Read the model definition and answer for the solid it produces. Units are mm, in the model's axes. Coordinates: 2 decimals unless noted, no trailing zeros. Order: outer loops, then holes, each group sorted by start corner. A loop starts at its lowest first (then second) coordinate and runs counter-clockwise, first axis right, second up.
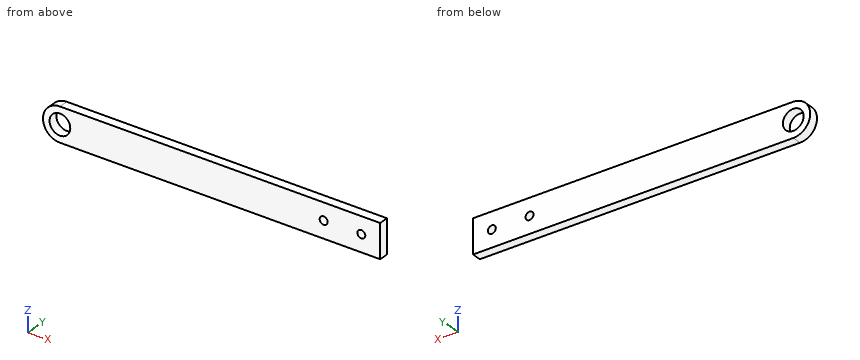
from build123d import *

# Parameters (mm, degrees)
BOSS_EXTRUDE1_DEPTH = 5
SKETCH4_R           = 2.1
CUT_EXTRUDE2_DEPTH  = 180.972220079
SKETCH5_R           = 5.5
CUT_EXTRUDE3_DEPTH  = 180.972220079


with BuildPart() as part:
    # Sketch1 → Boss-Extrude1 (new body)
    with BuildSketch(Plane(origin=(0, 0, 0), x_dir=(1, 0, 0), z_dir=(0, 1, 0))):
        with BuildLine():
            Line((0, 0), (-170, 0))
            ThreePointArc((-170, 0), (-179, -9), (-170, -18))
            Line((-170, -18), (0, -18))
            Line((0, -18), (0, 0))
        make_face()
    extrude(amount=BOSS_EXTRUDE1_DEPTH)

    # Sketch4 → Cut-Extrude2 (cut, through all)
    with BuildSketch(Plane(origin=(0, 5, 0), x_dir=(1, 0, 0), z_dir=(0, 1, 0))):
        with Locations(Location((-10, -9, 0), (0, 0, 270))):
            Circle(SKETCH4_R)
        with Locations(Location((-30, -9, 0), (0, 0, 270))):
            Circle(SKETCH4_R)
    extrude(amount=-CUT_EXTRUDE2_DEPTH, mode=Mode.SUBTRACT)

    # Sketch5 → Cut-Extrude3 (cut, through all)
    with BuildSketch(Plane(origin=(0, 5, 0), x_dir=(1, 0, 0), z_dir=(0, 1, 0))):
        with Locations(Location((-170, -9, 0), (0, 0, 270))):
            Circle(SKETCH5_R)
    extrude(amount=-CUT_EXTRUDE3_DEPTH, mode=Mode.SUBTRACT)


solid = part.part
Q1. The part is cut by section C-C, the plane z = 9. Determine the outline of the cut face in (x, y), then the cut area to 3 significant figures.
Q2. The part is cut by section B-B, the plane y = 3.5. Determine the outline of the cut face in (x, z).
Q3. The part is cut by section A-A, the plane x = -30. Determine the outline of the cut face in (y, z), then the cut area to 3 significant figures.
Q4. This flat-tipped pin is pushed along its axis until it touches: P1, Ø2.5, axis at x = -30, z = 9, coming from the -Y side. Where does it stop, or does it pass through?
Q5. Straight lines are drawn through the part: L1, parallel to X at y = 2, z = 9; L2, parallel to X at y = 3.25, z = 6.5; L3, parallel to Z at x = -168.5, y = 3.4. For each, find the intervals that lie inside material, in ascending order.
Computed values:
1. outline: (-179, 0) - (-175.5, 0) - (-175.5, 5) - (-179, 5) - close; (-164.5, 0) - (-32.1, 0) - (-32.1, 5) - (-164.5, 5) - close; (-27.9, 0) - (-12.1, 0) - (-12.1, 5) - (-27.9, 5) - close; (-7.9, 0) - (0, 0) - (0, 5) - (-7.9, 5) - close
1. area: 798 mm2
2. outline: (-170, 0) - (0, 0) - (0, 18) - (-170, 18) arc R9 ccw to start; hole circle Ø11 at (-170, 9); hole circle Ø4.2 at (-30, 9); hole circle Ø4.2 at (-10, 9)
3. outline: (0, 0) - (5, 0) - (5, 6.9) - (0, 6.9) - close; (0, 11.1) - (5, 11.1) - (5, 18) - (0, 18) - close
3. area: 69.0 mm2
4. P1: passes through
5. L1: x = -179 to -175.5, -164.5 to -32.1, -27.9 to -12.1, -7.9 to 0
5. L2: x = -178.65 to -174.9, -165.1 to 0
5. L3: z = 0 to 3.71, 14.29 to 18
